Can you work these out from the model? Positions are in its coordinate system, mm. A direction names the side the tool comes from. Round coordinates to 2 decimals unless told otherwise and drop trailing zeros. Write each loop counter-clockwise with the first axis right and the second up, starting at its lowest first coordinate (ties: lowest second). Pieces come first, ordered by that corner, then holes. Notation, with made-up numbers: M 30.25,34 L 82.25,34 A36 ccw 82.25,71 Z; hole C 80.25,52 d11. An arc over 180 degrees is marked long. Answer as a JSON object with one key per item and string values. Group by question number.
1) If we mould it in two halves opening along X, with no side actions, what happens to faces 1 (the flat face through (-10.5, 0, 3)), 2 (the flat face through (-17, 0, 6)), 3 (the flat face through (0, 17, 7))? For each: +X half, -X half, draft (parallel to the pull), parting line (faces both ways), or undercut.
2) Suppose I cut it at C-C, the plane y = -9. Write out the boundary of the cut face in (x, z).
3) Please list where these lines run through material, in increasing order: L1, parallel to Y at x = 0, z = 11; L2, parallel to X at y = 8, z = 2.5; L3, parallel to Z at x = 7.5, y = -7. Write a range as [from, to].
4) On a 3-axis mill with a long thin cutter (end or side, diameter ignored), from which of +Z, -Z, +X, -X, +Y, -Y can I reach the whole of each face in a straight line? I mean faces 4 (the flat face through (14, 0, 0)), 5 (the flat face through (0, 10.2, 10)), 6 (the flat face through (10.5, 0, 3)), 7 (the flat face through (17, 0, 6)), 8 (the flat face through (0, -10.2, 10)). Say none if no direction works.
5) Suppose I cut it at B-B, the plane y = 0. Write out the boundary of the cut face in (x, z).
6) Suppose I cut it at D-D, the plane x = -12. Write out the boundary of the cut face in (y, z), and give its area (3 significant figures).
7) I'm going to push flat-ended pins straight in: pin 1 Ø11 at (x, y) = (-2.5, -6.5) entering from -Z; pin 2 Ø2.5 at (x, z) = (-5.5, 10) entering from -Y; pin 3 Ø1 at (x, y) = (12.5, -12.5) entering from +Z. Where does each tip first touch, or does it pass through?
8) Suppose I cut it at A-A, the plane x = 0. Write out the boundary of the cut face in (y, z).
from build123d import *

# Parameters (mm, degrees)
F0_W        = 34
F0_H        = 34
F1_DEPTH    = 12.9
F2_W        = 21
F2_H        = 5.3
F3_DEPTH    = 34.001
F4_W        = 6.8
F4_H        = 4.8
F5_DEPTH    = 34.001
F6_R        = 8
F7_DEPTH    = 12.901
F8_R        = 7
F9_T1_DEPTH = 6.0500204163
F9_T3_DEPTH = 6.751561158


# Not quite as in the source:
# - a fillet or chamfer that OpenCascade refuses, or shapes differently, is made with other operations: its cross-section is extruded or revolved along the edge and cut away or added


with BuildPart() as f1:
    # F0 (on Top) → F1 (new body)
    with BuildSketch(Plane.XY):
        Rectangle(F0_W, F0_H)
    extrude(amount=F1_DEPTH)

    # F2 (on face) → F3 (cut, through all)
    with BuildSketch(Plane.XZ.offset(17)):
        with Locations((0, 2.65)):
            Rectangle(F2_W, F2_H)
    extrude(amount=-F3_DEPTH, mode=Mode.SUBTRACT)

    # F4 (on face) → F5 (cut, through all)
    with BuildSketch(Plane.YZ.offset(17)):
        with Locations((-13.6, 10.5)):
            Rectangle(F4_W, F4_H)
        with Locations((13.6, 10.5)):
            Rectangle(F4_W, F4_H)
    extrude(amount=-F5_DEPTH, mode=Mode.SUBTRACT)

    # F6 (on face) → F7 (cut, through all)
    with BuildSketch(Plane.XY.offset(12.9)):
        Circle(F6_R)
    extrude(amount=-F7_DEPTH, mode=Mode.SUBTRACT)

    # F8
    f8_edges = [f1.edges().sort_by_distance(p)[0] for p in [
        (17, -17, 4.05),
        (17, 17, 4.05),
        (-17, -17, 4.05),
        (-17, 17, 4.05),
    ]]
    fillet(f8_edges, radius=F8_R)

    # F9: fillet of radius 0.5 on 8 edges, made by hand

    # F9_s2 → F9_t1 (cut)
    with BuildSketch(Plane.XY.offset(8.1)):
        with BuildLine():
            ThreePointArc((17, -9.7), (16.8535533906, -10.0535533906), (16.5, -10.2))
            Line((16.5, -10.2), (16.5, -10.25))
            Line((16.5, -10.25), (16.9971422738, -10.25))
            Line((16.9971422738, -10.25), (17.0471218615, -10.2014285714))
            ThreePointArc((17.0471218615, -10.2014285714), (17.05, -10), (17.05, -9.7))
            Line((17.05, -9.7), (17, -9.7))
        make_face()
        with BuildLine():
            ThreePointArc((17, 9.7), (16.8535533906, 10.0535533906), (16.5, 10.2))
            Line((16.5, 10.2), (16.5, 10.25))
            Line((16.5, 10.25), (16.9971422738, 10.25))
            Line((16.9971422738, 10.25), (17.0471218615, 10.2014285714))
            ThreePointArc((17.0471218615, 10.2014285714), (17.05, 10), (17.05, 9.7))
            Line((17.05, 9.7), (17, 9.7))
        make_face()
        with BuildLine():
            ThreePointArc((-17, 9.7), (-16.8535533906, 10.0535533906), (-16.5, 10.2))
            Line((-16.5, 10.2), (-16.5, 10.25))
            Line((-16.5, 10.25), (-16.9971422738, 10.25))
            Line((-16.9971422738, 10.25), (-17.0471218615, 10.2014285714))
            ThreePointArc((-17.0471218615, 10.2014285714), (-17.05, 10), (-17.05, 9.7))
            Line((-17.05, 9.7), (-17, 9.7))
        make_face()
        with BuildLine():
            ThreePointArc((-17, -9.7), (-16.8535533906, -10.0535533906), (-16.5, -10.2))
            Line((-16.5, -10.2), (-16.5, -10.25))
            Line((-16.5, -10.25), (-16.9971422738, -10.25))
            Line((-16.9971422738, -10.25), (-17.0471218615, -10.2014285714))
            ThreePointArc((-17.0471218615, -10.2014285714), (-17.05, -10), (-17.05, -9.7))
            Line((-17.05, -9.7), (-17, -9.7))
        make_face()
    extrude(amount=F9_T1_DEPTH, mode=Mode.SUBTRACT)

    # F9_s4 → F9_t3 (cut)
    with BuildSketch(Plane.XY.offset(-1.451561158)):
        with BuildLine():
            ThreePointArc((11.0769230769, -16.9166636962), (10.6747781822, -16.802393552), (10.5, -16.4226162893))
            Line((10.5, -16.4226162893), (10.5, -16.9821200219))
            ThreePointArc((10.5, -16.9821200219), (10.789140501, -16.9553761415), (11.0769230769, -16.9166636962))
        make_face()
        with BuildLine():
            ThreePointArc((-11.0769230769, -16.9166636962), (-10.6747781822, -16.802393552), (-10.5, -16.4226162893))
            Line((-10.5, -16.4226162893), (-10.5, -16.9821200219))
            ThreePointArc((-10.5, -16.9821200219), (-10.789140501, -16.9553761415), (-11.0769230769, -16.9166636962))
        make_face()
        with BuildLine():
            ThreePointArc((-11.0769230769, 16.9166636962), (-10.6747781822, 16.802393552), (-10.5, 16.4226162893))
            Line((-10.5, 16.4226162893), (-10.5, 16.9821200219))
            ThreePointArc((-10.5, 16.9821200219), (-10.789140501, 16.9553761415), (-11.0769230769, 16.9166636962))
        make_face()
        with BuildLine():
            ThreePointArc((11.0769230769, 16.9166636962), (10.6747781822, 16.802393552), (10.5, 16.4226162893))
            Line((10.5, 16.4226162893), (10.5, 16.9821200219))
            ThreePointArc((10.5, 16.9821200219), (10.789140501, 16.9553761415), (11.0769230769, 16.9166636962))
        make_face()
    extrude(amount=F9_T3_DEPTH, mode=Mode.SUBTRACT)


solid = f1.part
Results:
{
 "1": {"face 1": "undercut", "face 2": "-X half", "face 3": "draft"},
 "2": {"outline": "M -17,0 L -10.5,0 L -10.5,5.3 L 10.5,5.3 L 10.5,0 L 17,0 L 17,12.9 L -17,12.9 Z"},
 "3": {"L1": "[-10.2, -8], [8, 10.2]", "L2": "[-17, -10.5], [10.5, 17]", "L3": "[5.3, 12.9]"},
 "4": {"face 4": "-Z, +X, -X, +Y, -Y", "face 5": "+Z, +X, -X, +Y", "face 6": "-Z, +Y, -Y", "face 7": "+Z, -Z, +X, +Y, -Y", "face 8": "+Z, +X, -X, -Y"},
 "5": {"outline": "M -17,0 L -10.5,0 L -10.5,5.3 L -8,5.3 L -8,12.9 L -17,12.9 Z; M 8,5.3 L 10.5,5.3 L 10.5,0 L 17,0 L 17,12.9 L 8,12.9 Z"},
 "6": {"outline": "M -16.71,0 L 16.71,0 L 16.71,8.1 L 10.2,8.1 L 10.2,12.9 L -10.2,12.9 L -10.2,8.1 L -16.71,8.1 Z", "area": "369 mm^2"},
 "7": {"pin 1": "z = 5.3", "pin 2": "y = -10.2", "pin 3": "z = 8.1"},
 "8": {"outline": "M -17,5.3 L -8,5.3 L -8,12.9 L -10.2,12.9 L -10.2,8.1 L -17,8.1 Z; M 8,5.3 L 17,5.3 L 17,8.1 L 10.2,8.1 L 10.2,12.9 L 8,12.9 Z"}
}
